Check sheet for the modelled part. Datum: model origin and axes. Units: mm. A direction names the side the tool comes from. Round coordinates to 2 decimals unless told otherwise and drop trailing zeros. Loops run counter-clockwise (first coordinate to the right, second up) from the corner with the lowest first, then second, coordinate; pieces in that order, holes last. Notation, with made-up numbers: M -31.5,-7 L 4.5,-7 A22 ccw 4.5,21 Z; hole C 48.5,23 d2. An arc over 180 degrees is marked long. Write item = value, one per line. Start each with the question number.
(1) Cross-section at A-A on x = 0. Record the boundary of the cut face in (y, z), plus the area to 3 significant figures.
(2) Cross-section at D-D on y = -12. Record the boundary of the cut face in (x, z).
(3) Cross-section at C-C on x = -10.25. Record the boundary of the cut face in (y, z), plus the area to 3 significant figures.
(4) Cross-section at B-B on z = 3.5. Record the boundary of the cut face in (x, y) (3 decimals), plus the area to 3 significant figures.
(5) Mould release check, pull along X, two halves, no side actions. Record for faces 1 (the face through (0, 4, 0)), 2 (the face through (-5.388, -3.167, 4.437)), 3 (the face through (9.11, 3.114, 4.437)), 4 (the face through (-14.985, 0.66, 4.437)): pulls with the +X half, pulls with the -X half, needs draft (parallel to the pull), parting line crosses it, or undercut.
(6) Set-up check for faces 5 (the face through (5.44, -3.08, 4.44)), 6 (the face through (0, 4, 9)): record each of +Z, -Z, +X, -X, +Y, -Y from which the full face is reachable in a straight line by a thin tool's end or side.
(7) Go/stop test with flat-tipped pins: P1, Ø4, axis at x = 11.5, z = 2, coming from the -Y side; P2, Ø3, axis at y = 5, z = 3, coming from the +X side. Record where each tip stops, or that it passes through.
(8) Scan lines: L1, parallel to Y at x = 0, z = 6; L2, parallel to X at y = -0.25, z = 5.75 (3 decimals); L3, parallel to X at y = -1.75, z = 6. Record each from-to range of solid material in increasing order. Write a range as from..to.
from build123d import *

# Parameters (mm, degrees)
SKETCH_1_R      = 15
SKETCH_1_R_2    = 3.25
EXTRUDE_1_DEPTH = 9


with BuildPart() as part:
    # 草图1 → 凸台-拉伸1 (new body)
    with BuildSketch(Plane.XY):
        Circle(SKETCH_1_R)
        Circle(SKETCH_1_R_2, mode=Mode.SUBTRACT)
        with BuildLine():
            ThreePointArc((6.269982777, 10.231681972), (0, 12), (-6.269982777, 10.231681972))
            ThreePointArc((-6.269982777, 10.231681972), (-7.219139876, 6.278158126), (-3.265616029, 5.329001027))
            ThreePointArc((-3.265616029, 5.329001027), (0, 6.25), (3.265616029, 5.329001027))
            ThreePointArc((3.265616029, 5.329001027), (7.219139876, 6.278158126), (6.269982777, 10.231681972))
        make_face(mode=Mode.SUBTRACT)
        with BuildLine():
            ThreePointArc((5.725905123, -10.545805352), (10.392304845, -6), (11.9958879, 0.31412338))
            ThreePointArc((11.9958879, 0.31412338), (9.046614364, 3.112879463), (6.247858281, 0.163605927))
            ThreePointArc((6.247858281, 0.163605927), (5.412658774, -3.125), (2.982242252, -5.492606954))
            ThreePointArc((2.982242252, -5.492606954), (1.827474488, -9.391037589), (5.725905123, -10.545805352))
        make_face(mode=Mode.SUBTRACT)
        with BuildLine():
            ThreePointArc((-11.9958879, 0.31412338), (-10.392304845, -6), (-5.725905123, -10.545805352))
            ThreePointArc((-5.725905123, -10.545805352), (-1.827474488, -9.391037589), (-2.982242252, -5.492606954))
            ThreePointArc((-2.982242252, -5.492606954), (-5.412658774, -3.125), (-6.247858281, 0.163605927))
            ThreePointArc((-6.247858281, 0.163605927), (-9.046614364, 3.112879463), (-11.9958879, 0.31412338))
        make_face(mode=Mode.SUBTRACT)
    extrude(amount=EXTRUDE_1_DEPTH)


solid = part.part
Result:
q1.outline = M -15,0 L -3.25,0 L -3.25,9 L -15,9 Z; M 3.25,0 L 6.25,0 L 6.25,9 L 3.25,9 Z; M 12,0 L 15,0 L 15,9 L 12,9 Z
q1.area = 160 mm^2
q2.outline = M -9,0 L 9,0 L 9,9 L -9,9 Z
q3.outline = M -10.95,0 L -6.24,0 L -6.24,9 L -10.95,9 Z; M 2.88,0 L 10.95,0 L 10.95,9 L 2.88,9 Z
q3.area = 115 mm^2
q4.outline = C 0,0 d30; hole M -11.996,0.314 A12 ccw -5.726,-10.546 A2.875 ccw -2.982,-5.493 A6.25 cw -6.248,0.164 A2.875 ccw Z; hole M -6.27,10.232 A2.875 ccw -3.266,5.329 A6.25 cw 3.266,5.329 A2.875 ccw 6.27,10.232 A12 ccw Z; hole C 0,0 d6.5; hole M 2.982,-5.493 A2.875 ccw 5.726,-10.546 A12 ccw 11.996,0.314 A2.875 ccw 6.248,0.164 A6.25 cw Z
q4.area = 423 mm^2
q5.face_1 = needs draft
q5.face_2 = undercut
q5.face_3 = undercut
q5.face_4 = parting line crosses it
q6.face_5 = +Z, -Z
q6.face_6 = +Z, +X, -X, +Y, -Y
q7.P1 = -11.61
q7.P2 = 14.59
q8.L1 = -15..-3.25, 3.25..6.25, 12..15
q8.L2 = -14.998..-11.997, -6.245..-3.24, 3.24..6.245, 11.997..14.998
q8.L3 = -14.9..-11.87, -6..-2.74, 2.74..6, 11.87..14.9
